Geometry: see drawing. Coordinates: mm, zero at the bounding-box minimum. Round coordinates to 2 decimals unless told otherwise and drop trailing zeros. Order: outer loops, then holes, each group sorted by start corner. A loop starts at its lowest first (then second) coordinate and runs counter-clockwise, first axis right, second up. Notation, with made-up numbers: (39, 45.5) - (45, 45.5) arc R24 cw to (45, 77.5) - close; hole circle Ø9 at (57.5, 17.5). An arc over 180 degrees is marked (long way). Put each result on its own line as item: value. Start each with the question number.
1) Section C-C on z = 9.5. Output: boundary loops of the cut face in (x, y), then the cut area to 3 significant figures.
2) Line query: probe 1 along Y at (x, z) = (3.5, 22); probe 2 along X at (y, z) = (7, 71); probe 3 along X at (y, z) = (1.5, 10.5). Output: solid intervals per line, ascending. Write a range as [from, to].
3) Section B-B on z = 74. Output: boundary loops of the cut face in (x, y).
4) Section A-A on x = 3.5. Output: boundary loops of the cut face in (y, z).
5) Contact query for flat-ended pins moving along their axis: P1, Ø1, axis at y = 7, z = 51.5, coming from the -X side; P2, Ø0.6, axis at y = 7, z = 46.5, coming from the +X side; P3, Ø1.5, axis at y = 6.5, z = 54.5, coming from the -X side. Output: stop coordinate, or through.
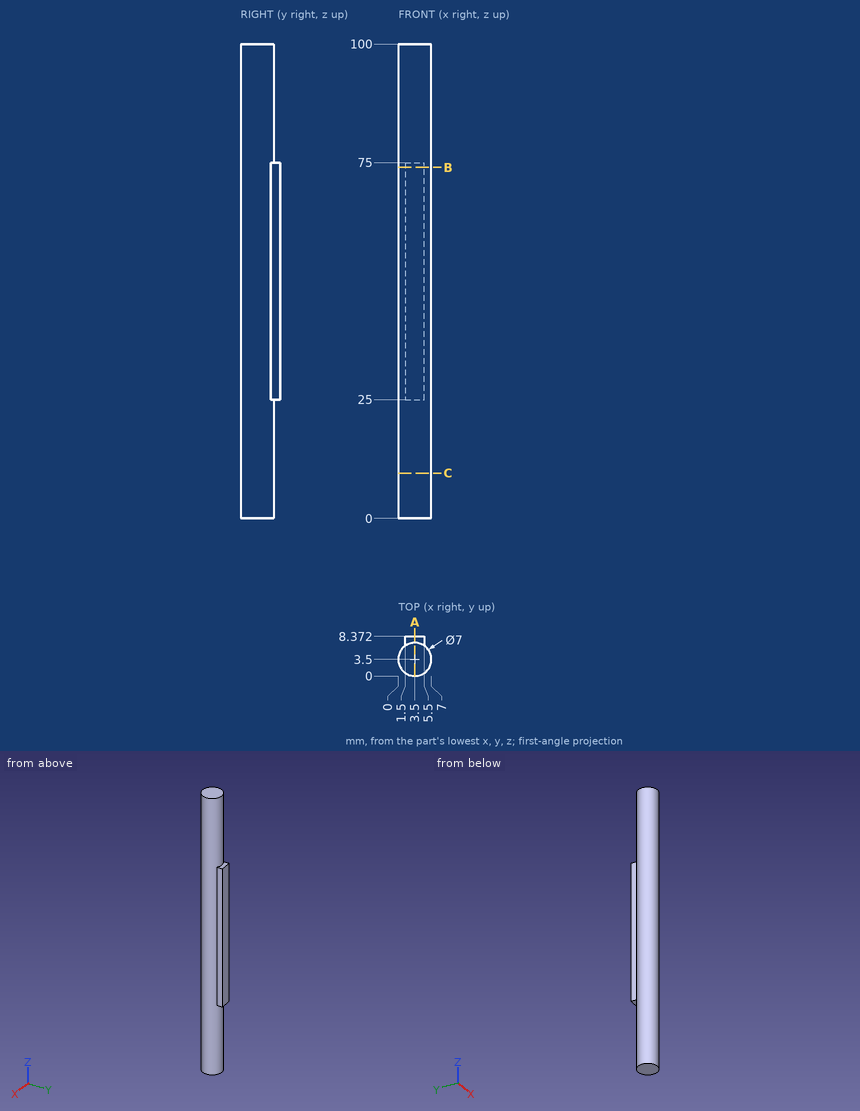
Answer sheet:
1. outline: circle Ø7 at (3.5, 3.5)
1. area: 38.5 mm^2
2. probe 1: [0, 7]
2. probe 2: [1.5, 5.5]
2. probe 3: [0.63, 6.37]
3. outline: (1.5, 6.37) arc R3.5 ccw (long way) to (5.5, 6.37) - (5.5, 8.37) - (1.5, 8.37) - close
4. outline: (0, 0) - (7, 0) - (7, 25) - (8.37, 25) - (8.37, 75) - (7, 75) - (7, 100) - (0, 100) - close
5. P1: x = 1.5
5. P2: x = 5.5
5. P3: x = 0.82
